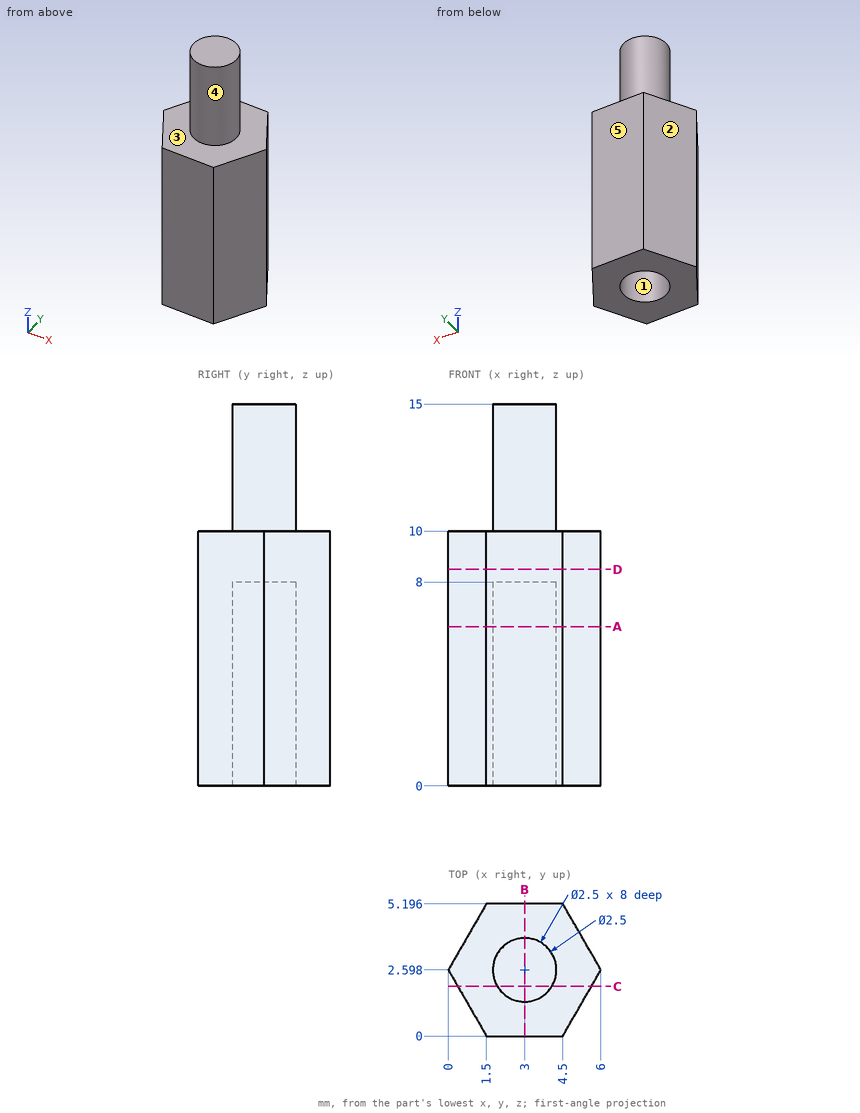
For this review, use the dimensioned drawing (mm, ordinates from the lowest corner) and the shaded views. A direction names the side the tool comes from. Give positions to 0.01 mm unless a question says otherwise; leave off trailing zeros. Loops run counter-clockwise (first coordinate to the right, second up) from the corner with the lowest first, then second, coordinate; pieces in that order, holes last.
Item 1: Insertion check: pin 1 (2 mm diameter, centred on x = 2, y = 3, fed in from -Z); pin 2 (2 mm diameter, centred on x = 3, y = 2.6, fed in from -Z); pin 3 (1 mm diameter, centred on y = 1, z = 7, fed in from -X); pin 4 (1.5 mm diameter, centred on x = 4, z = 12, fed in from -Y). Each pin has a flat end and moves straight along its axis. Give the tip position at first contact, or say it passes through.
Item 2: For line 1 along Y through (x, z) = (3, 3); line 2 along Z through (x, y) = (3.6, 0.75); line 3 along Y through (x, z) = (3.3, 5.75) (1 decimal), list the stretches that pass through material, from the lowest coordinate up.
Item 3: Take a section at C-C, the plane y = 1.95. State the section outline as (x, z) points.
Item 4: Take a section at A-A, the plane z = 6.25. State the section outline as (x, y) points, and give its area (3 significant figures).
Item 5: Tool access review of the marked faces 4 and 5: name each direction out of +Z, -Z, +X, -X, +Y, -Y from which nothing blocks a thin tool from reaching the whole face with its end or side.
Item 6: Take a section at D-D, the plane z = 8.5. State the section outline as (x, y) points, and give its area (3 significant figures).
Item 7: Take a section at B-B, the plane x = 3. State the section outline as (y, z) points.
Item 8: Draft analysis for pull direction Y (two halves, no side actions). For the marked faces 1, 2 and 3, state which applies: +Y half, -Y half, draft (parallel to the pull), parting line (faces both ways), or undercut.
Calculated:
1. pin 1: stops at z = 0
1. pin 2: stops at z = 8
1. pin 3: stops at x = 0.63
1. pin 4: stops at y = 1.37
2. line 1: y = 0 to 1.35, 3.85 to 5.2
2. line 2: z = 0 to 10
2. line 3: y = 0 to 1.4, 3.8 to 5.2
3. outline: (0.37, 0) - (1.93, 0) - (1.93, 8) - (4.07, 8) - (4.07, 0) - (5.63, 0) - (5.63, 10) - (4.07, 10) - (4.07, 15) - (1.93, 15) - (1.93, 10) - (0.37, 10) - close
4. outline: (0, 2.6) - (1.5, 0) - (4.5, 0) - (6, 2.6) - (4.5, 5.2) - (1.5, 5.2) - close; hole circle Ø2.5 at (3, 2.6)
4. area: 18.5 mm2
5. face 4: +Z
5. face 5: +Z, -Z, +X, -X, +Y
6. outline: (0, 2.6) - (1.5, 0) - (4.5, 0) - (6, 2.6) - (4.5, 5.2) - (1.5, 5.2) - close
6. area: 23.4 mm2
7. outline: (0, 0) - (1.35, 0) - (1.35, 8) - (3.85, 8) - (3.85, 0) - (5.2, 0) - (5.2, 10) - (3.85, 10) - (3.85, 15) - (1.35, 15) - (1.35, 10) - (0, 10) - close
8. face 1: undercut
8. face 2: +Y half
8. face 3: draft
